Build history of the part. All positions in model axes, mm. A direction names the side the tool comes from. Round coordinates to 2 decimals unless told otherwise and drop trailing zeros. Write each loop counter-clockwise with the first axis right and the second up, starting at its lowest first coordinate (ties: lowest second). Pieces come first, ordered by that corner, then holes. Notation, with made-up numbers: M 61,14.25 L 87,14.25 A12 cw 87,25.25 Z; hole C 68.25,63.25 d9. An arc over 180 degrees is marked long. One line per item, written item: value. Start each with the question number.
```python
from build123d import *

# Parameters (mm, degrees)
ESQUISSE1_W             = 13
ESQUISSE1_H             = 13
BOSS_EXTRU_1_DEPTH      = 5.6
ESQUISSE2_W             = 9
ESQUISSE2_H             = 13
ENL_V_MAT_EXTRU_1_DEPTH = 3.6
ESQUISSE3_R             = 2.1
ENL_V_MAT_EXTRU_2_DEPTH = 10.872183143
ESQUISSE4_W             = 13
ESQUISSE4_H             = 13
BOSS_EXTRU_2_DEPTH      = 3
CONG_1_R                = 1


with BuildPart() as part:
    # Esquisse1 → Boss.-Extru.1 (new body)
    with BuildSketch(Plane.XY):
        Rectangle(ESQUISSE1_W, ESQUISSE1_H)
    extrude(amount=BOSS_EXTRU_1_DEPTH)

    # Esquisse2 → Enlèv. mat.-Extru.1 (cut)
    with BuildSketch(Plane.XY.offset(5.6)):
        Rectangle(ESQUISSE2_W, ESQUISSE2_H)
    extrude(amount=-ENL_V_MAT_EXTRU_1_DEPTH, mode=Mode.SUBTRACT)

    # Esquisse3 → Enlèv. mat.-Extru.2 (cut, through all)
    with BuildSketch(Plane.XY.offset(2)):
        Circle(ESQUISSE3_R)
    extrude(amount=-ENL_V_MAT_EXTRU_2_DEPTH, mode=Mode.SUBTRACT)

    # Esquisse4 → Boss.-Extru.2 (add)
    with BuildSketch(Plane(origin=(0, 0, 0), x_dir=(-1, 0, 0), z_dir=(0, 0, -1))):
        Rectangle(ESQUISSE4_W, ESQUISSE4_H)
        Polygon((-3.75, -2.165063509), (0, -4.330127019), (3.75, -2.165063509), (3.75, 2.165063509), (0, 4.330127019), (-3.75, 2.165063509), align=None, mode=Mode.SUBTRACT)
    extrude(amount=BOSS_EXTRU_2_DEPTH)

    # Congé1
    cong_1_edges = [part.edges().sort_by_distance(p)[0] for p in [
        (6.5, 0, -3),
        (0, -6.5, -3),
        (-6.5, 0, -3),
        (0, 6.5, -3),
    ]]
    fillet(cong_1_edges, radius=CONG_1_R)


solid = part.part
```
Item 1: Which spindle directions (+Z, -Z, +X, -X, +Y, -Y) get a long thin tool onto all of the face, cutting with end or side? Do faces 4 (the cylindrical face through (6.215, 0.091, -2.699)), 5 (the flat face through (1.901, -3.232, -1.479)), 6 (the flat face through (-4.5, 0, 4)). Say none if no direction does.
Item 2: Drill centre lines: line 1 (X direction, y = 3.25, z = 5); line 2 (Y direction, x = 0, z = 1.45); line 3 (Z direction, x = -1.25, y = 2). Where is each one in solid material? Low to high.
Item 3: Cut at A-A, the plane z = 2.5. Write the cut outline in (x, y).
Item 4: Drop flat-ended pins along their axis: pin 1 (5.5 mm diameter, centred on x = 0, y = 0, fed in from +Z); pin 2 (4 mm diameter, centred on x = 1, y = 0, fed in from -Z). Give the stop position or say it passes through.
Item 5: Cut at D-D, the plane x = 1. Write the cut outline in (y, z).
Item 6: Cut at C-C, the plane y = 0. Write the cut outline in (x, z), plus the area to 3 significant figures.
Item 7: Cut at B-B, the plane z = -0.25. Write the cut outline in (x, y), plus the area to 3 significant figures.
Item 8: Two-plate mould, pull along Y, no slides. Class faces 1 (the cylindrical face through (2.003, 0.631, 1.014)), 2 (the cylindrical face through (-0.091, 6.215, -2.699)), 3 (the flat face through (5, 0, 5.6)): pulls with the +Y half, pulls with the -Y half, needs draft (parallel to the pull), parting line crosses it, or undercut.
Computed values:
1. face 4: -Z, +X, +Y, -Y
1. face 5: -Z
1. face 6: +Z, +Y, -Y
2. line 1: x = -6.5 to -4.5, 4.5 to 6.5
2. line 2: y = -6.5 to -2.1, 2.1 to 6.5
2. line 3: z = 0 to 2
3. outline: M -6.5,-6.5 L -4.5,-6.5 L -4.5,6.5 L -6.5,6.5 Z; M 4.5,-6.5 L 6.5,-6.5 L 6.5,6.5 L 4.5,6.5 Z
4. pin 1: stops at z = 2
4. pin 2: stops at z = 0
5. outline: M -6.5,-2 A1 ccw -5.5,-3 L -3.75,-3 L -3.75,0 L -1.85,0 L -1.85,2 L -6.5,2 Z; M 1.85,0 L 3.75,0 L 3.75,-3 L 5.5,-3 A1 ccw 6.5,-2 L 6.5,2 L 1.85,2 Z
6. outline: M -6.5,-2 A1 ccw -5.5,-3 L -3.75,-3 L -3.75,0 L -2.1,0 L -2.1,2 L -4.5,2 L -4.5,5.6 L -6.5,5.6 Z; M 2.1,0 L 3.75,0 L 3.75,-3 L 5.5,-3 A1 ccw 6.5,-2 L 6.5,5.6 L 4.5,5.6 L 4.5,2 L 2.1,2 Z
6. area: 48.1 mm2
7. outline: M -6.5,-6.5 L 6.5,-6.5 L 6.5,6.5 L -6.5,6.5 Z; hole M -3.75,-2.17 L 0,-4.33 L 3.75,-2.17 L 3.75,2.17 L 0,4.33 L -3.75,2.17 Z
7. area: 120 mm2
8. face 1: undercut
8. face 2: pulls with the +Y half
8. face 3: needs draft
